Part model, mm, in its own coordinate system. A direction names the side the tool comes from. Coordinates: 2 decimals unless noted, no trailing zeros. Loops run counter-clockwise (first coordinate to the right, second up) from the corner with the lowest first, then second, coordinate; pieces in that order, holes last.
```python
from build123d import *

# Parameters (mm, degrees)
F0_W     = 69.85
F0_H     = 12.7
F0_W_2   = 63.5
F0_H_2   = 7.62
F1_DEPTH = 5.08
F2_R     = 1.26999


# Not quite as in the source:
# - a fillet or chamfer is up to 0.001 mm smaller than in the source, because OpenCascade refuses the exact size


with BuildPart() as f1:
    # F0 (on Top) → F1 (new body)
    with BuildSketch(Plane.XY):
        Rectangle(F0_W, F0_H)
        Rectangle(F0_W_2, F0_H_2, mode=Mode.SUBTRACT)
    extrude(amount=F1_DEPTH)

    # F2 (radius 1.27 in the source; OpenCascade refuses exactly that, so slightly less here)
    f2_edges = [f1.edges().sort_by_distance(p)[0] for p in [
        (0, 6.35, 5.08),
        (-34.925, 0, 5.08),
        (0, -6.35, 5.08),
        (34.925, 0, 5.08),
        (-31.75, 0, 5.08),
        (0, 3.81, 5.08),
        (31.75, 0, 5.08),
        (0, -3.81, 5.08),
        (0, 6.35, 0),
        (-34.925, 0, 0),
        (0, -6.35, 0),
        (34.925, 0, 0),
        (-31.75, 0, 0),
        (0, 3.81, 0),
        (31.75, 0, 0),
        (0, -3.81, 0),
    ]]
    fillet(f2_edges, radius=F2_R)


solid = f1.part
```
Q1. Drop flat-ended pins along their axis: P1, Ø5, axis at x = -12, y = -2.5, coming from the +Z side; P2, Ø2, axis at x = 17.5, y = 3, coming from the -Z side. Give the stop position or say it passes through.
Q2. Tool access for faces 1 (the cylindrical face through (-32.112, 0.071, 4.698)), 2 (the cylindrical face through (0.462, -4.172, 0.382)), 3 (the flat face through (0, -3.81, 3)): list every direction of +Z, -Z, +X, -X, +Y, -Y with a clear straight run to the whole face (end or side of a thin tool).
Q3. Mould opens along X. For faces 4 (the flat face through (0, 3.81, 3)), 5 (the flat face through (34.925, 0, 3)), 6 (the flat face through (0, -6.35, 3)), 7 (the cylindrical face through (32.112, 0.071, 4.698)) say: released by +X, released by -X, zero draft, split by the parting line, or undercut.
Q4. Saw through at C-C (z = 2.45). List the corners of the cut face in (x, y) (3 decimals), plus the area to 3 significant figures.
Q5. Saw through at A-A (y = 0). List the corners of the cut face in (x, z) (3 decimals).
Q6. Probe line 1 (Y direction, x = -25, z = 3.9); line 2 (X direction, y = -1.25, z = 1.6) (3 decimals). List the from-to ranges inside material, lowest first.
Checked values:
1. P1: stops at z = 5.08
1. P2: stops at z = 0.6
2. face 1: +Z
2. face 2: -Z
2. face 3: +Z, -Z
3. face 4: undercut
3. face 5: released by +X
3. face 6: zero draft
3. face 7: undercut
4. outline: (-34.925, -6.35) - (34.925, -6.35) - (34.925, 6.35) - (-34.925, 6.35) - close; hole (-31.75, -3.81) - (31.75, -3.81) - (31.75, 3.81) - (-31.75, 3.81) - close
4. area: 403 mm2
5. outline: (-34.925, 1.27) arc R1.27 ccw to (-33.655, 0) - (-33.02, 0) arc R1.27 ccw to (-31.75, 1.27) - (-31.75, 3.81) arc R1.27 ccw to (-33.02, 5.08) - (-33.655, 5.08) arc R1.27 ccw to (-34.925, 3.81) - close; (31.75, 1.27) arc R1.27 ccw to (33.02, 0) - (33.655, 0) arc R1.27 ccw to (34.925, 1.27) - (34.925, 3.81) arc R1.27 ccw to (33.655, 5.08) - (33.02, 5.08) arc R1.27 ccw to (31.75, 3.81) - close
6. line 1: y = -6.35 to -3.81, 3.81 to 6.35
6. line 2: x = -34.925 to -31.75, 31.75 to 34.925
